from build123d import *

# Parameters (mm, degrees)
EXTRUDE_1_DEPTH     = 98
EXTRUDE_2_DEPTH     = 25
SKETCH_4_R          = 16.45
EXTRUDE_6_DEPTH     = 14.3
SKETCH_5_R          = 15
EXTRUDE_7_DEPTH     = 5
SKETCH_6_R          = 16
EXTRUDE_8_DEPTH     = 23
SKETCH_7_R          = 5
CUT_EXTRUDE_2_DEPTH = 5
HOLE_WIZARD_M5_1_D  = 4.2


with BuildPart() as part:
    # Sketch 1 → Extrude 1 (new body)
    with BuildSketch(Plane.XY):
        Polygon((0, 0), (0, 133), (8, 133), (8, 5), (92, 5), (92, 0), align=None)
    extrude(amount=EXTRUDE_1_DEPTH)



with BuildPart() as body_2:
    # Sketch 2 → Extrude 2 (new, symmetric)
    with BuildSketch(Plane.XY.offset(49)):
        Polygon((66.16, 36), (64.16, 36), (64.16, 38), (63.16, 38), (63.16, 59), (53.16, 59), (19.5, 51), (19.5, 5), (66.16, 5), align=None)
    extrude(amount=EXTRUDE_2_DEPTH, both=True)


with BuildPart() as part_1:
    add(part.part)

    add(body_2.part)  # Extrude 6 merges body 2
    # Sketch 4 → Extrude 6 (add)
    with BuildSketch(Plane(origin=(66.16, 0, 0), x_dir=(0, 0, -1), z_dir=(1, 0, 0))):
        with Locations(Location((-49, 21.5, 0), (0, 0, 118.181138406))):
            Circle(SKETCH_4_R)
    extrude(amount=EXTRUDE_6_DEPTH)

    # Sketch 5 → Extrude 7 (add)
    with BuildSketch(Plane(origin=(-10.430514532, 43.886389891, 0), x_dir=(0.9728991739264884, 0.23122975019049047, 0), z_dir=(-0.23122975019049047, 0.9728991739264884, 0))):
        with Locations(Location((48.063063249, -49, 0), (0, 0, 180))):
            Circle(SKETCH_5_R)
    extrude(amount=EXTRUDE_7_DEPTH)

    # Sketch 6 → Extrude 8 (add)
    with BuildSketch(Plane(origin=(-11.586663283, 48.750885761, 0), x_dir=(0.9728991739264884, 0.2312297501904905, 0), z_dir=(-0.2312297501904905, 0.9728991739264884, 0))):
        with Locations(Location((48.063063249, -49, 0), (0, 0, 180))):
            Circle(SKETCH_6_R)
    extrude(amount=EXTRUDE_8_DEPTH)

    # Sketch 7 → Cut-Extrude 2 (cut)
    with BuildSketch(Plane(origin=(0, 0, 24), x_dir=(-1, 0, 0), z_dir=(0, 0, -1))):
        with Locations((-50.16, 21)):
            Circle(SKETCH_7_R)
    extrude(amount=-CUT_EXTRUDE_2_DEPTH, mode=Mode.SUBTRACT)

    # Hole Wizard M5 _1 (through all)
    with Locations(Plane.ZY):
        with Locations((24, 63), (49, 63), (74, 63), (74, 88), (49, 88), (24, 88), (24, 113), (49, 113), (74, 113)):
            Hole(HOLE_WIZARD_M5_1_D / 2)


solid = part_1.part
The model under review builds one solid part; all positions refer to its coordinate system, in mm. A direction names the side the tool comes from. Round coordinates to 2 decimals unless told otherwise and drop trailing zeros. Loops run counter-clockwise (first coordinate to the right, second up) from the corner with the lowest first, then second, coordinate; pieces in that order, holes last. Notation, with made-up numbers: M 2,1 L 21,1 A27 ccw 21,37 Z; hole C 28.5,4.25 d7. An arc over 180 degrees is marked long. Answer as CSV lines item,"result". Start each with the question number.
Item 1: Consider section A-A (y = 88). Write out the cut boundary in (x, z).
Item 2: Consider section C-C (y = 9.5). Write out the cut boundary in (x, z).
Item 3: Mouldability with a two-part tool opening along Z and no side actions: class faces 4 (the face through (5, 47, 0)), 5 (the face through (51.526, 58.612, 49.35)), 6 (the face through (4.056, 86.137, 23.031)) as released by +Z, released by -Z, zero draft, split by the parting line, or undercut.
Item 4: Insertion check: P1, Ø15.5, axis at y = 13, z = 45, coming from the +X side; P2, Ø2, axis at x = 19, z = 72, coming from the +Y side; P3, Ø11, axis at x = 48.5, y = 23, coming from the -Z side; P4, Ø3.5, axis at y = 88, z = 74, coming from the +X side. Each pin has a flat end and moves straight along its axis. Give the tip position at first contact, or say it passes through.
Item 5: For faces 1 (the face through (63.16, 48, 49)), 2 (the face through (43, 32, 74)), 3 (the face through (30.1, 82.3, 49.2)), list the 3-axis set-ups (+Z, -Z, +X, -X, +Y, -Y) from which the entire face can be reached by the end or side of a thin tool; tool diameter is ignored.
Item 6: Consider section B-B (x = 69). Write out the cut boundary in (y, z).
Item 7: Consider section D-D (z = 14). Write out the cut boundary in (x, y), then the cut area to 3 significant figures.
Item 8: Wall thickness on line 1 (Y direction, x = 2, z = 74); line 2 (X direction, y = 9, z = 30); line 3 (X direction, y = 16, z = 61): over which ranges is each line inside the solid? List them lowest first. Write a range as [from, to].
Answer:
1,outline,"M 0,0 L 8,0 L 8,21.9 L 0,21.9 Z; M 0,26.1 L 8,26.1 L 8,46.9 L 0,46.9 Z; M 0,51.1 L 8,51.1 L 8,71.9 L 0,71.9 Z; M 0,76.1 L 8,76.1 L 8,98 L 0,98 Z"
2,outline,"M 0,0 L 8,0 L 8,98 L 0,98 Z; M 19.5,24 L 66.16,24 L 66.16,37.75 L 80.46,37.75 L 80.46,60.25 L 66.16,60.25 L 66.16,74 L 19.5,74 Z"
3,face 4,"released by -Z"
3,face 5,"zero draft"
3,face 6,"undercut"
4,P1,"stops at x = 80.46"
4,P2,"stops at y = 51.12"
4,P3,"stops at z = 24"
4,P4,"passes through"
5,face 1,"+Z, -Z, +X, +Y"
5,face 2,"+Z, +X, +Y"
5,face 3,"+Z, -Z, +Y"
6,outline,"M 0,0 L 5,0 L 5,98 L 0,98 Z; C 21.5,49 d32.9"
7,outline,"M 0,0 L 92,0 L 92,5 L 8,5 L 8,133 L 0,133 Z"
7,area,"1,480 mm^2"
8,line 1,"y = [0, 60.9], [65.1, 85.9], [90.1, 110.9], [115.1, 133]"
8,line 2,"x = [0, 8], [19.5, 66.16]"
8,line 3,"x = [0, 8], [19.5, 80.46]"
